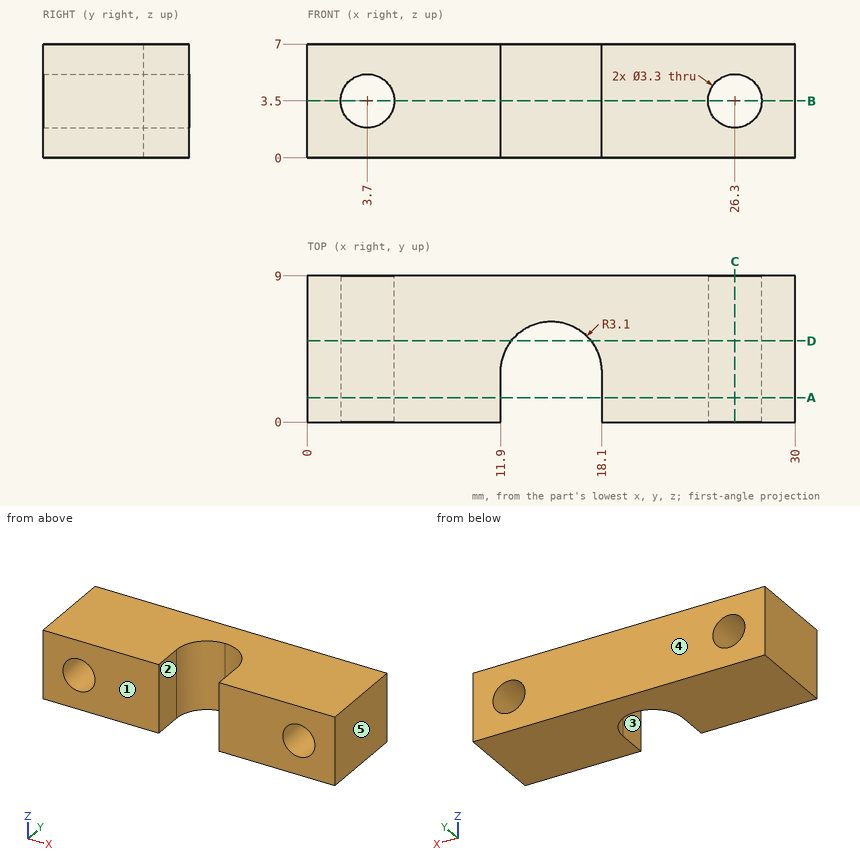
Drawing for the job (mm, zero at the part's lowest x, y, z). A direction names the side the tool comes from. Round coordinates to 2 decimals unless told otherwise and drop trailing zeros. Loops run counter-clockwise (first coordinate to the right, second up) from the corner with the lowest first, then second, coordinate; pieces in that order, holes last. Notation, with made-up numbers: M -9.5,-27 L 21.5,-27 A5 cw 21.5,-18 Z; hole C -2,-20 d6. An arc over 180 degrees is marked long. Use a Markdown table: item, result. Add a question column.
(1) Cut at D-D (y = 5). Give the cut face in (x, z), and give its area (3 significant figures).
(2) Which spindle directions (+Z, -Z, +X, -X, +Y, -Y) get a long thin tool onto all of the face, cutting with end or side? Do the marked faces 1 and 2. Say none if no direction does.
(3) Cut at B-B (z = 3.5). Give the cut face in (x, y).
(4) Pull direction X, two halves, no side cores. Call the marked faces 3, 4 and 5: +X half, -X half, draft (parallel to the pull), parting line (faces both ways), or undercut.
(5) Drill centre lines: line 1 (Z direction, x = 26.3, y = 5); line 2 (X direction, y = 3.25, z = 1.5); line 3 (X direction, y = 7, z = 3.25). Where is each one in solid material? Low to high.
(6) Cut at C-C (x = 26.3). Give the cut face in (y, z), and give its area (3 significant figures).
(7) Cut at A-A (y = 1.5). Give the cut face in (x, z), and give its area (3 significant figures).
Geometry says:
| question | item | result |
|---|---|---|
| 1 | outline | M 0,0 L 12.55,0 L 12.55,7 L 0,7 Z; M 17.45,0 L 30,0 L 30,7 L 17.45,7 Z; hole C 3.7,3.5 d3.3; hole C 26.3,3.5 d3.3 |
| 1 | area | 159 mm² |
| 2 | face 1 | +Z, -Z, +X, -X, -Y |
| 2 | face 2 | +Z, -Z, -Y |
| 3 | outline | M 0,0 L 2.05,0 L 2.05,9 L 0,9 Z; M 5.35,0 L 11.9,0 L 11.9,3.1 A3.1 cw 18.1,3.1 L 18.1,0 L 24.65,0 L 24.65,9 L 5.35,9 Z; M 27.95,0 L 30,0 L 30,9 L 27.95,9 Z |
| 4 | face 3 | undercut |
| 4 | face 4 | draft |
| 4 | face 5 | +X half |
| 5 | line 1 | z = 0 to 1.85, 5.15 to 7 |
| 5 | line 2 | x = 0 to 11.9, 18.1 to 30 |
| 5 | line 3 | x = 0 to 2.07, 5.33 to 24.67, 27.93 to 30 |
| 6 | outline | M 0,0 L 9,0 L 9,1.85 L 0,1.85 Z; M 0,5.15 L 9,5.15 L 9,7 L 0,7 Z |
| 6 | area | 33.3 mm² |
| 7 | outline | M 0,0 L 11.9,0 L 11.9,7 L 0,7 Z; M 18.1,0 L 30,0 L 30,7 L 18.1,7 Z; hole C 3.7,3.5 d3.3; hole C 26.3,3.5 d3.3 |
| 7 | area | 149 mm² |
